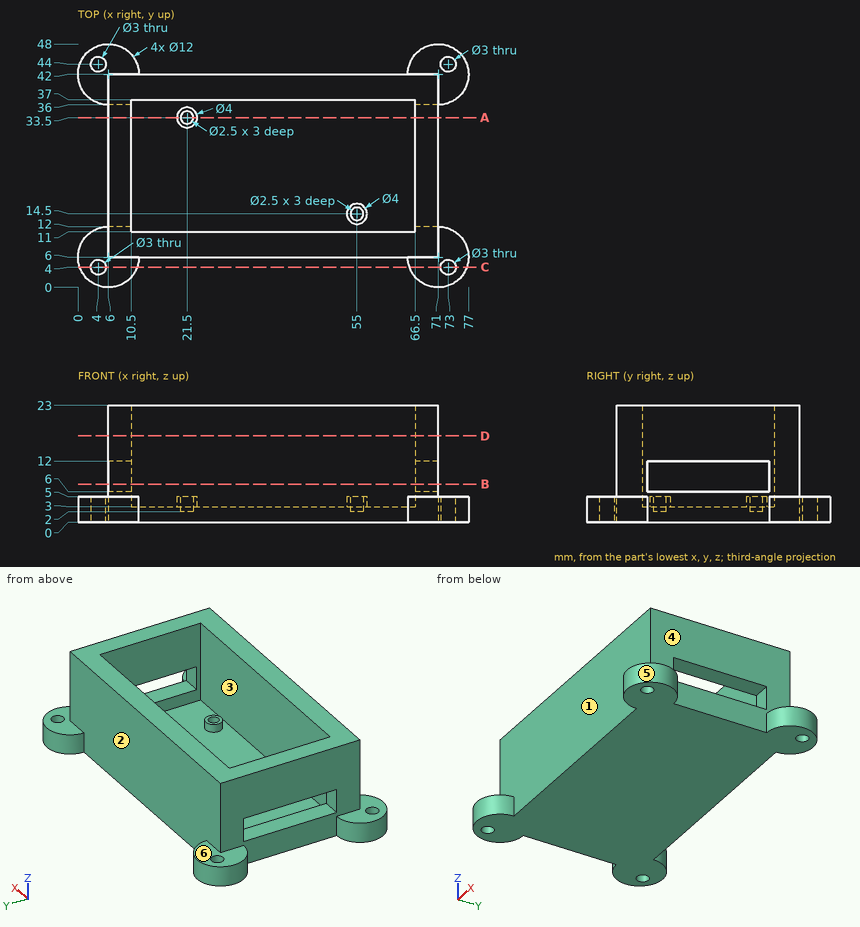
Study the drawing (mm; zero at the part's minimum x, y, z) and answer. A direction names the side the tool comes from. Round coordinates to 2 decimals unless told otherwise and drop trailing zeros. Write each loop counter-clockwise with the first axis right and the second up, starting at its lowest first coordinate (ties: lowest second). Pieces come first, ordered by that corner, then holes. Notation, with made-up numbers: (28.25, 84.25) - (44.25, 84.25) arc R19 cw to (44.25, 105.25) - close; hole circle Ø10 at (42, 83.25). An arc over 180 degrees is marked (long way). Use a Markdown table: item, result. Add a question column.
1. For a pull along X with two mould halves and no side action, classify the marked faces 4, 5 and 6 as +X half, -X half, draft (parallel to the pull), parting line (faces both ways), or undercut.
2. The part is cut by section B-B (z = 7.5). Write down the section's boundary in (x, y), and give its area (3 significant figures).
3. The part is cut by section D-D (z = 17). Write down the section's boundary in (x, y), and give its area (3 significant figures).
4. Consider line 1 (Y direction, x = 21.5, z = 4.2); line 2 (X direction, y = 18, z = 17.5); line 3 (Y direction, x = 7.5, z = 11.75). Determine where each line is inside the solid, lowest interval first.
5. The part is cut by section C-C (y = 4). Write down the section's boundary in (x, z).
6. The part is cut by section A-A (y = 33.5). Write down the section's boundary in (x, z), and give its area (4 significant figures).
7. A tool of negligible diameter and unlimited length cuts with its end or side. For the marked faces 1, 2 and 3, from which of +Z, -Z, +X, -X, +Y, -Y can it reach the whole face along a straight path? Write none if from no direction.
8. Flat-ended cylindrical pins translate along their axes: P1, Ø10, axis at x = 13, z = 14.5, coming from the +Y side; P2, Ø2, axis at x = 54.5, y = 14.5, coming from the +Z side; P3, Ø5, axis at x = 57, y = 28, coming from the +Z side; P4, Ø2.5, axis at x = 4, y = 44, coming from the +Z side. Find the tip coordinate at first contact, or state that the pin passes through.
Reported:
| question | item | result |
|---|---|---|
| 1 | face 4 | +X half |
| 1 | face 5 | undercut |
| 1 | face 6 | draft |
| 2 | outline | (6, 6) - (71, 6) - (71, 12) - (66.5, 12) - (66.5, 11) - (10.5, 11) - (10.5, 12) - (6, 12) - close; (6, 36) - (10.5, 36) - (10.5, 37) - (66.5, 37) - (66.5, 36) - (71, 36) - (71, 42) - (6, 42) - close |
| 2 | area | 668 mm^2 |
| 3 | outline | (6, 6) - (71, 6) - (71, 42) - (6, 42) - close; hole (10.5, 11) - (66.5, 11) - (66.5, 37) - (10.5, 37) - close |
| 3 | area | 884 mm^2 |
| 4 | line 1 | 6 to 11, 31.5 to 32.25, 34.75 to 35.5, 37 to 42 |
| 4 | line 2 | 6 to 10.5, 66.5 to 71 |
| 4 | line 3 | 6 to 12, 36 to 42 |
| 5 | outline | (0.34, 0) - (2.5, 0) - (2.5, 5) - (0.34, 5) - close; (5.5, 0) - (11.66, 0) - (11.66, 5) - (5.5, 5) - close; (65.34, 0) - (71.5, 0) - (71.5, 5) - (65.34, 5) - close; (74.5, 0) - (76.66, 0) - (76.66, 5) - (74.5, 5) - close |
| 6 | outline | (6, 0) - (71, 0) - (71, 6) - (66.5, 6) - (66.5, 3) - (23.5, 3) - (23.5, 5) - (22.75, 5) - (22.75, 2) - (20.25, 2) - (20.25, 5) - (19.5, 5) - (19.5, 3) - (10.5, 3) - (10.5, 6) - (6, 6) - close; (6, 12) - (10.5, 12) - (10.5, 23) - (6, 23) - close; (66.5, 12) - (71, 12) - (71, 23) - (66.5, 23) - close |
| 6 | area | 321.5 mm^2 |
| 7 | face 1 | +Z, -Y |
| 7 | face 2 | +Z, +Y |
| 7 | face 3 | +Z |
| 8 | P1 | y = 42 |
| 8 | P2 | z = 5 |
| 8 | P3 | z = 3 |
| 8 | P4 | through |
